from build123d import *
from build123d.topology import SkipClean

# Parameters (mm, degrees)
SKIZZE1_R                       = 2.5
AUFSATZ_LINEAR_AUSTRAGEN1_DEPTH = 5
AUFSATZ_LINEAR_START            = 7
AUFSATZ_LINEAR_AUSTRAGEN2_DEPTH = 7
AUFSATZ_LINEAR_START_2          = 3
SKIZZE3_R                       = 6
AUFSATZ_LINEAR_AUSTRAGEN3_DEPTH = 3
BOSS_EXTRUDE1_START             = 3
BOSS_EXTRUDE1_DEPTH             = 3


with BuildPart() as part:
    # Skizze1 → Aufsatz-Linear austragen1 (new body)
    with BuildSketch(Plane.XY):
        with BuildLine():
            ThreePointArc((-6.068344121, -3.48929787), (3.48929787, -6.068344121), (6.068344121, 3.48929787))
            Line((6.068344121, 3.48929787), (-1.366900012, 16.420157233))
            ThreePointArc((-1.366900012, 16.420157233), (-7.048924024, 12.258998302), (-13.503588255, 9.441561493))
            Line((-13.503588255, 9.441561493), (-6.068344121, -3.48929787))
        make_face()
        Circle(SKIZZE1_R, mode=Mode.SUBTRACT)
    extrude(amount=AUFSATZ_LINEAR_AUSTRAGEN1_DEPTH)

    # Skizze2 → Aufsatz-Linear austragen2 (add)
    with BuildSketch(Plane(origin=(0, 0, 0), x_dir=(-1, 0, 0), z_dir=(0, 0, -1)).offset(AUFSATZ_LINEAR_START)):
        with BuildLine():
            Line((8.518877013, 0.772498463), (13.503588255, 9.441561493))
            ThreePointArc((13.503588255, 9.441561493), (7.048924023, 12.258998302), (1.366900012, 16.420157232))
            Line((1.366900012, 16.420157233), (-3.61781123, 7.751094202))
            Line((-3.61781123, 7.751094202), (8.518877013, 0.772498463))
        make_face()
    extrude(amount=-AUFSATZ_LINEAR_AUSTRAGEN2_DEPTH)

    # Skizze3 → Aufsatz-Linear austragen3 (add)
    with BuildSketch(Plane(origin=(0, 0, -7), x_dir=(-1, 0, 0), z_dir=(0, 0, -1)).offset(AUFSATZ_LINEAR_START_2)):
        with BuildLine():
            Line((1.366900012, 16.420157233), (-3.61781123, 7.751094202))
            Line((-3.61781123, 7.751094202), (8.518877013, 0.772498463))
            Line((8.518877013, 0.772498463), (13.503588255, 9.441561493))
            ThreePointArc((13.503588255, 9.441561493), (13.684230172, 9.386009203), (13.865197027, 9.331524742))
            Line((13.865197027, 9.331524742), (30.209148043, 35.496869479))
            ThreePointArc((30.209148043, 35.496869479), (27.237004556, 47.368703576), (15.481560492, 43.965232321))
            Line((15.481560492, 43.965232321), (1.089891738, 16.677325284))
            ThreePointArc((1.089891738, 16.677325284), (1.228016167, 16.548332256), (1.366900012, 16.420157233))
        make_face()
        with Locations((23, 40)):
            Circle(SKIZZE3_R, mode=Mode.SUBTRACT)
    extrude(amount=-AUFSATZ_LINEAR_AUSTRAGEN3_DEPTH)

    # Sketch1 → Boss-Extrude1 (add)
    with SkipClean():  # the faces are left unmerged after this step: merging them gives an invalid solid
        with BuildSketch(Plane(origin=(0, 0, -10), x_dir=(-1, 0, 0), z_dir=(0, 0, -1)).offset(BOSS_EXTRUDE1_START)):
            with BuildLine():
                ThreePointArc((24.687363033, 31.669165348), (27.842500084, 33.014286512), (30.209148043, 35.496869479))
                Line((30.209148043, 35.496869479), (28.088810383, 36.821319632))
                ThreePointArc((28.088810383, 36.821319632), (27.694055373, 36.262909667), (27.238322861, 35.753045877))
                Line((27.238322861, 35.753045877), (24.687363033, 31.669165348))
            make_face()
            with BuildLine():
                Line((13.865197027, 9.331524742), (30.209148043, 35.496869479))
                ThreePointArc((30.209148043, 35.496869479), (27.842500084, 33.014286512), (24.687363033, 31.669165348))
                Line((24.687363033, 31.669165348), (6.215378123, 2.097010324))
                Line((6.215378123, 2.097010324), (8.518877013, 0.772498463))
                Line((8.518877013, 0.772498463), (13.503588255, 9.441561493))
                ThreePointArc((13.503588255, 9.441561493), (13.684230172, 9.386009203), (13.865197027, 9.331524742))
            make_face()
            with BuildLine():
                Line((28.088810383, 36.821319632), (30.209148043, 35.496869479))
                ThreePointArc((30.209148043, 35.496869479), (31.170916667, 37.657753041), (31.5, 40))
                ThreePointArc((31.5, 40), (25.342246959, 48.170916667), (15.790851957, 44.503130521))
                Line((15.790851957, 44.503130521), (17.911189617, 43.178680368))
                ThreePointArc((17.911189617, 43.178680368), (24.653350795, 45.767705883), (29, 40))
                ThreePointArc((29, 40), (28.767705883, 38.346649205), (28.088810383, 36.821319632))
            make_face()
            with BuildLine():
                Line((17.911189617, 43.178680368), (15.790851957, 44.503130521))
                Line((15.790851957, 44.503130521), (15.216048877, 43.414689578))
                ThreePointArc((15.216048877, 43.414689578), (14.507527777, 40.35765281), (14.956507243, 37.25186895))
                Line((14.956507243, 37.25186895), (17.181735723, 41.465537717))
                ThreePointArc((17.181735723, 41.465537717), (17.479602927, 42.350577834), (17.911189617, 43.178680368))
            make_face()
            with BuildLine():
                Line((-1.32040378, 6.430084919), (14.956507243, 37.25186895))
                ThreePointArc((14.956507243, 37.25186895), (14.507527777, 40.35765281), (15.216048877, 43.414689578))
                Line((15.216048877, 43.414689578), (1.094048415, 16.673421058))
                ThreePointArc((1.094048415, 16.673421058), (1.230105912, 16.546392359), (1.366900012, 16.420157233))
                Line((1.366900012, 16.420157233), (-3.61781123, 7.751094202))
                Line((-3.61781123, 7.751094202), (-1.32040378, 6.430084919))
            make_face()
        extrude(amount=-BOSS_EXTRUDE1_DEPTH)


solid = part.part
Verification items for the finished model (mm, model axes). A direction names the side the tool comes from. Give positions to 0.01 mm unless a question says otherwise; leave off trailing zeros. Write each loop counter-clockwise with the first axis right and the second up, starting at its lowest first coordinate (ties: lowest second). Pieces come first, ordered by that corner, then holes. Notation, with made-up numbers: (18.25, -5.5) -> (34.25, -5.5) arc R19 cw to (34.25, 9.5) -> close; hole circle Ø11 at (36.25, 37). An arc over 180 degrees is marked (long way). Use CSV: the item, a comma, the result in double quotes.
(1) Release check for a two-part mould opening along X. For faces 4 (the cylindrical face through (3.36, -6.14, 2.46)), 5 (the flat face through (-10, 28.3, -13)), 6 (the flat face through (-12, 20, -10)) record: +X half, -X half, draft (parallel to the pull), parting line (faces both ways), or undercut.
Derived:
face 4,"parting line"
face 5,"draft"
face 6,"undercut"
(2) Set-up check for faces 1 (the flat face through (-16, 29, -7)), 2 (the cylindrical face through (-0.54, -2.44, 2.46)), 3 (the flat face through (1, -3, 0)): record each of +Z, -Z, +X, -X, +Y, -Y from which the full face is reachable in a straight line by a thin tool's end or side.
Derived:
face 1,"+Z, -X, +Y"
face 2,"+Z, -Z"
face 3,"-Z, +X, -Y"
(3) Go/stop test with flat-tipped pins: pin 1 (3 mm diameter, centred on x = -6, z = -0.5, fed in from +Y); pin 2 (5 mm diameter, centred on y = 42.5, z = -5, fed in from -X); pin 3 (6 mm diameter, centred on x = -14.5, y = 24, fed in from -Z); pin 4 (11 mm diameter, centred on x = -23, y = 40, fed in from -Z). Record where each tip stops, or that it passes through.
Derived:
pin 1,"stops at y = 13.89"
pin 2,"stops at x = -31.44"
pin 3,"stops at z = -10"
pin 4,"passes through"
(4) Sectioned sample at B-B (x = -22). Record the cut outline in (y, z), plus the area to 3 significant figures.
Derived:
outline,"(22.35, -13) -> (27.37, -13) -> (27.37, -10) -> (34.08, -10) -> (34.08, -7) -> (22.35, -7) -> close; (45.92, -13) -> (48.44, -13) -> (48.44, -7) -> (45.92, -7) -> close"
area,"65.4 mm^2"
(5) Material ranges on L1, parallel to Y at x = 0, z = 3.3; L2, parallel to Y at x = -23, z = -9.1; L3, parallel to Z at x = -7, y = 0.5, recorded low to high.
Derived:
L1,"y = -7 to -2.5, 2.5 to 14.04"
L2,"y = 23.96 to 34, 46 to 48.5"
L3,"z = 0 to 5"
(6) Sectioned sample at A-A (y = 0). Record the cut outline in (x, z).
Derived:
outline,"(-8.07, 0) -> (-2.5, 0) -> (-2.5, 5) -> (-8.07, 5) -> close; (2.5, 0) -> (7, 0) -> (7, 5) -> (2.5, 5) -> close"
(7) Sectioned sample at C-C (x = 0). Record the cut outline in (y, z), plus the area to 3 significant figures.
Derived:
outline,"(-7, 0) -> (-2.5, 0) -> (-2.5, 5) -> (-7, 5) -> close; (2.5, 0) -> (5.67, 0) -> (5.67, -10) -> (8.93, -10) -> (8.93, -13) -> (14.04, -13) -> (14.04, 5) -> (2.5, 5) -> close"
area,"179 mm^2"
